Verification items for the finished model (mm, model axes). A direction names the side the tool comes from. Coordinates: 2 decimals unless noted, no trailing zeros. Order: outer loops, then holes, each group sorted by start corner. A loop starts at its lowest first (then second) coordinate and runs counter-clockwise, first axis right, second up. Notation, with made-up numbers: M 39.5,68.5 L 91.5,68.5 A13 ccw 91.5,76.5 Z; hole C 43,17 d1. An arc over 180 degrees is marked long. Return JSON: item names as keys, results as strings. Group by question number.
1. Mould release check, pull along X, two halves, no side actions. Record for faces 3 (the flat face through (2, 5, 0)), 4 (the cylindrical face through (-1.73, 7.81, -0.76)), 5 (the cylindrical face through (6.8, 0, -0.8)): +X half, -X half, draft (parallel to the pull), parting line (faces both ways), or undercut.
2. Section check A-A, the plane x = 0. Give the number of separate pieces and of enclosed holes in the cut face, plus the area to 3 significant figures.
3. Material ranges on line 1 along Y through (x, z) = (0, -0.75); line 2 along Z through (x, y) = (-4.5, -4.5); line 3 along Y through (x, z) = (0, 3.5), recorded low to high.
4. Section check C-C, the plane x = 6. Record the cut outline in (y, z).
5. Gauge pin test, flat ends, axial feed: pin 1 (1.3 mm diameter, centred on x = 6, y = 0, fed in from +Z); pin 2 (1 mm diameter, centred on y = -4, z = 4.5, fed in from +X); pin 3 (2 mm diameter, centred on x = 3.5, z = 0.5, fed in from +Y); pin 4 (2 mm diameter, centred on x = 5.5, z = 2.5, fed in from -Y). Record the tip position at first contact, or that the pin passes through.
6. Set-up check for faces 1 (the cylindrical face through (-1.08, -4.88, 2.96)), 2 (the flat face through (0, 2, -1.5)): record each of +Z, -Z, +X, -X, +Y, -Y from which the full face is reachable in a straight line by a thin tool's end or side.
```python
from build123d import *

# Parameters (mm, degrees)
SKETCH1_R               = 5
BOSS_EXTRUDE1_DEPTH     = 6
SKETCH2_R               = 8
BOSS_EXTRUDE2_DEPTH     = 1.5
BOSS_EXTRUDE3_START     = 1.5
SKETCH3_R               = 8
BOSS_EXTRUDE3_DEPTH     = 1.5
CUT_EXTRUDE1_DEPTH      = 15.456832295
CUT_EXTRUDE1_DEPTH_BACK = 15.456832295
SKETCH4_R               = 0.8
CUT_EXTRUDE2_DEPTH      = 15.456832295
CUT_EXTRUDE2_DEPTH_BACK = 15.456832295
SKETCH5_R               = 1


with BuildPart() as part:
    # Sketch1 → Boss-Extrude1 (new body)
    with BuildSketch(Plane.XY):
        Circle(SKETCH1_R)
    extrude(amount=BOSS_EXTRUDE1_DEPTH)

    # Sketch2 → Boss-Extrude2 (add)
    with BuildSketch(Plane.XY.offset(6)):
        Circle(SKETCH2_R)
    extrude(amount=BOSS_EXTRUDE2_DEPTH)

    # Sketch3 → Boss-Extrude3 (add)
    with BuildSketch(Plane(origin=(0, 0, 0), x_dir=(-1, 0, 0), z_dir=(0, 0, -1)).offset(BOSS_EXTRUDE3_START)):
        with Locations(Location((0, 0, 0), (0, 0, 180))):
            Circle(SKETCH3_R)
    extrude(amount=-BOSS_EXTRUDE3_DEPTH)

    # Sketch4 → Cut-Extrude1 (cut, two sides: drawn at the far end of the back side and taken through both)
    with BuildSketch(Plane.XY.offset(7.5).offset(-CUT_EXTRUDE1_DEPTH_BACK)):
        with Locations((-6, 0)):
            Circle(SKETCH4_R)
        with Locations(Location((6, 0, 0), (0, 0, 180))):
            Circle(SKETCH4_R)
        with Locations((0, 6)):
            Circle(SKETCH4_R)
        with Locations(Location((0, -6, 0), (0, 0, 180))):
            Circle(SKETCH4_R)
    extrude(amount=CUT_EXTRUDE1_DEPTH + CUT_EXTRUDE1_DEPTH_BACK, mode=Mode.SUBTRACT)

    # Sketch5 → Cut-Extrude2 (cut, two sides: drawn at the far end of the back side and taken through both)
    with BuildSketch(Plane.XY.offset(7.5).offset(-CUT_EXTRUDE2_DEPTH_BACK)):
        Circle(SKETCH5_R)
    extrude(amount=CUT_EXTRUDE2_DEPTH + CUT_EXTRUDE2_DEPTH_BACK, mode=Mode.SUBTRACT)


solid = part.part
```
Answers follow:
{
 "1": {"face 3": "draft", "face 4": "parting line", "face 5": "undercut"},
 "2": {"separate pieces": "6", "enclosed holes": "0", "area": "80.4 mm^2"},
 "3": {"line 1": "-8 to -6.8, -5.2 to -1, 1 to 5.2, 6.8 to 8", "line 2": "-1.5 to 0, 6 to 7.5", "line 3": "-5 to -1, 1 to 5"},
 "4": {"outline": "M -5.29,-1.5 L -0.8,-1.5 L -0.8,0 L -5.29,0 Z; M -5.29,6 L -0.8,6 L -0.8,7.5 L -5.29,7.5 Z; M 0.8,-1.5 L 5.29,-1.5 L 5.29,0 L 0.8,0 Z; M 0.8,6 L 5.29,6 L 5.29,7.5 L 0.8,7.5 Z"},
 "5": {"pin 1": "through", "pin 2": "x = 3.57", "pin 3": "y = 7.55", "pin 4": "y = -2.18"},
 "6": {"face 1": "none", "face 2": "-Z, +X, -X, +Y, -Y"}
}
